Source: CAD feature listing. Evaluate the final solid. Frame: model axes, mm. Face numbers are marked on the shaded views. A direction names the side the tool comes from. Coordinates: 2 decimals unless noted, no trailing zeros. Order: outer loops, then holes, each group sorted by start corner. A loop starts at its lowest first (then second) coordinate and runs counter-clockwise, first axis right, second up.
Item 1: Section B-B on x = 0. Return the cut outline in (y, z).
Item 2: Contact query for flat-ended pins moving along their axis: P1, Ø10, axis at x = -66, y = -50.5, coming from the +Z side; P2, Ø12, axis at x = -33.5, y = 19.5, coming from the +Z side; P3, Ø1, axis at x = 70.5, y = 13.5, coming from the +Z side. Output: stop coordinate, or through.
Item 3: Section C-C on z = 0. Return the cut outline in (x, y), then the cut area to 3 significant figures.
Item 4: Reachability of the marked faces 1 and 2 from +Z, -Z, +X, -X, +Y, -Y: full face, straight path, thin tool, end or side. Return the list, or none.
Item 5: Ray query, line 1 (X direction, y = -1.5, z = -90); line 2 (Z direction, x = 37, y = 14.5); line 3 (X direction, y = -65, z = 45). Return the intervals inside material, ascending.
Item 6: Section A-A on y = 0. Return the cut outline in (x, z), then the cut area to 3 significant figures.
Item 7: Section D-D on z = -79.5. Return the cut outline in (x, y), then the cut area to 3 significant figures.
Autodesk Inventor part; units mm, degrees
ref_plane "YZ Plane" through (0, 0, 0) normal (1, 0, 0) x (0, 1, 0)
sketch "スケッチ1" plane through (0, 0, 0) normal (0, 0, 1) x (1, 0, 0)
  arc A0 (0, 90) -> (0, -90) centre (0, 0) ccw
  line L0 (0, 90) -> (0, -90)
  dimension "d0" = 180
revolve "回転1" add sketch "スケッチ1" angle 360 about axis through (0, 90, 0) along (0, -1, 0)
sketch "スケッチ2" plane through (0, 0, 0) normal (0, 1, 0) x (-1, 0, 0)
  circle A0 centre (0, 0) radius 20
  dimension "d2" = 40
extrude "押し出し1" add sketch "スケッチ2" along normal mid plane 200
sketch "スケッチ3" plane through (0, 0, 0) normal (0, 0, 1) x (1, 0, 0)
  circle A0 centre (0, 0) radius 50
  dimension "d5" = 100
extrude "押し出し2" add sketch "スケッチ3" against normal blind 100
chamfer "面取り1" distance 5 angle 45 1 edges at (-50, 0, -100)
properties part number "ChestY"
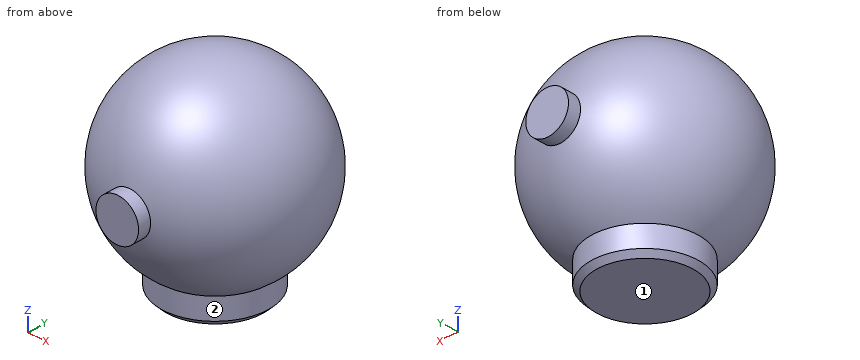
Answer list:
1. outline: (-100, -20) - (-87.75, -20) arc R90 ccw to (-50, -74.83) - (-50, -95) - (-45, -100) - (45, -100) - (50, -95) - (50, -74.83) arc R90 ccw to (87.75, -20) - (100, -20) - (100, 20) - (87.75, 20) arc R90 ccw to (-87.75, 20) - (-100, 20) - close
2. P1: stops at z = 44.72
2. P2: stops at z = 83.83
2. P3: stops at z = 54.95
3. outline: (-20, -100) - (20, -100) - (20, -87.75) arc R90 ccw to (20, 87.75) - (20, 100) - (-20, 100) - (-20, 87.75) arc R90 ccw to (-20, -87.75) - close
3. area: 26,300 mm2
4. face 1: -Z, +X, -X, +Y, -Y
4. face 2: -Z
5. line 1: x = -49.98 to 49.98
5. line 2: z = -100 to 80.75
5. line 3: x = -43.01 to 43.01
6. outline: (-50, -95) - (-45, -100) - (45, -100) - (50, -95) - (50, -74.83) arc R90 ccw (long way) to (-50, -74.83) - close
6. area: 26,900 mm2
7. outline: circle Ø100 at (0, 0)
7. area: 7,850 mm2
